Could you check a few things on this model? Use its own coordinates, in mm. A direction names the side the tool comes from. Round coordinates to 2 decimals unless told otherwise and drop trailing zeros. Write each loop counter-clockwise with the first axis right and the second up, starting at its lowest first coordinate (ties: lowest second). Pieces come first, ordered by that corner, then holes. Notation, with made-up numbers: (43.5, 49) -> (62.5, 49) arc R8 cw to (62.5, 59) -> close; hole circle Ø1 at (43, -9). An arc over 180 degrees is marked (long way). Answer as CSV lines item,"result". Start each with the question number.
Q1. Imagine slicing it at A-A on x = -4.5. Please give me the cut outline in (y, z).
Q2. For faces 1 (the flat face through (-2.932, -0.393, 2.761)), 2 (the cylindrical face through (-3.3, 1.41, -15.44)), 3 (the flat face through (0, 0.9, 3)), 4 (the flat face through (0, -0.9, 3)), 5 (the flat face through (0, 1.95, -15)), which set-ups out of +Z, -Z, +X, -X, +Y, -Y let a thin tool reach every point of the face, with its end or its side?
Q3. Imagine slicing it at B-B on y = 3. Please give me the cut outline in (x, z).
Q4. Will these pins go through, and if not, where does the flat tip stop? pin 1 Ø1.5 at (x, y) = (-4.5, -3) entering from +Z; pin 2 Ø2.5 at (x, z) = (0.5, -15) entering from +Y.
Q5. If I drill on line 1 (X direction, y = 0.5, z = 0.5) (3 decimals); line 2 (Z direction, x = -4, y = 0); line 3 (Y direction, x = -2, z = 3), over which ranges is the centre line in solid material (lowest first)? Write a range as [from, to].
from build123d import *

# Parameters (mm, degrees)
SKETCH1_W           = 11
SKETCH1_H           = 8.5
BOSS_EXTRUDE1_DEPTH = 14
SKETCH2_W           = 7.75
SKETCH2_H           = 3.9
BOSS_EXTRUDE2_DEPTH = 2.85
SKETCH4_W           = 6.85
SKETCH4_H           = 1.8
BOSS_EXTRUDE4_DEPTH = 5.6
FILLET6_R           = 0.3
CHAMFER1_SIZE       = 1
CUT_EXTRUDE1_DEPTH  = 0.15
CIRPATTERN1_COUNT   = 2
FILLET1_R           = 1.9
FILLET3_R           = 0.75
FILLET4_R           = 0.75


with BuildPart() as part:
    # Sketch1 → Boss-Extrude1 (new body)
    with BuildSketch(Plane.XY):
        Rectangle(SKETCH1_W, SKETCH1_H)
    extrude(amount=-BOSS_EXTRUDE1_DEPTH)

    # Sketch2 → Boss-Extrude2 (add)
    with BuildSketch(Plane(origin=(0, 0, -14), x_dir=(-1, 0, 0), z_dir=(0, 0, -1))):
        Rectangle(SKETCH2_W, SKETCH2_H)
    extrude(amount=BOSS_EXTRUDE2_DEPTH)

    # Sketch4 → Boss-Extrude4 (add)
    with BuildSketch(Plane.XY):
        Rectangle(SKETCH4_W, SKETCH4_H)
    extrude(amount=BOSS_EXTRUDE4_DEPTH)

    # Fillet6
    fillet6_edges = [part.edges().sort_by_distance(p)[0] for p in [
        (3.425, 0.9, 2.8),
        (-3.425, 0.9, 2.8),
    ]]
    fillet(fillet6_edges, radius=FILLET6_R)

    # Chamfer1
    chamfer1_edges = [part.edges().sort_by_distance(p)[0] for p in [
        (3.425, -0.9, 2.8),
        (-3.425, -0.9, 2.8),
    ]]
    chamfer(chamfer1_edges, length=CHAMFER1_SIZE)

    # Sketch5 → Cut-Extrude1 (cut)
    with BuildSketch(Plane.XZ.offset(4.25)):
        with BuildLine():
            Line((0, -3.279495805), (-0.485840634, -4.214842566))
            Line((-0.485840634, -4.214842566), (-0.093629021, -4.214842566))
            Line((-0.093629021, -4.214842566), (-0.093629021, -7.363659965))
            Line((-0.093629021, -7.363659965), (-1.035027967, -6.623865099))
            ThreePointArc((-1.035027967, -6.623865099), (-1.082535613, -6.564943154), (-1.099509752, -6.491182388))
            Line((-1.099509752, -6.491182388), (-1.099509752, -6.225332236))
            ThreePointArc((-1.099509752, -6.225332236), (-1.214270304, -5.348067145), (-1.329030856, -6.225332236))
            Line((-1.329030856, -6.225332236), (-1.329030856, -6.428798928))
            ThreePointArc((-1.329030856, -6.428798928), (-1.278108438, -6.650081225), (-1.135585502, -6.82684706))
            Line((-1.135585502, -6.82684706), (-0.158110806, -7.59499192))
            ThreePointArc((-0.158110806, -7.59499192), (-0.11060316, -7.653913865), (-0.093629021, -7.727674631))
            Line((-0.093629021, -7.727674631), (-0.093629021, -8.098323238))
            ThreePointArc((-0.093629021, -8.098323238), (0, -9.291083784), (0.093629021, -8.098323238))
            Line((0.093629021, -8.098323238), (0.093629021, -7.087908213))
            ThreePointArc((0.093629021, -7.087908213), (0.116268533, -7.003479025), (0.178112432, -6.941703889))
            Line((0.178112432, -6.941703889), (1.273368459, -6.310440139))
            ThreePointArc((1.273368459, -6.310440139), (1.458900155, -6.12511473), (1.526818691, -5.871827167))
            Line((1.526818691, -5.871827167), (1.526818691, -5.55143287))
            Line((1.526818691, -5.55143287), (1.774241614, -5.55143287))
            Line((1.774241614, -5.55143287), (1.774241614, -4.840448102))
            Line((1.774241614, -4.840448102), (1.063256846, -4.840448102))
            Line((1.063256846, -4.840448102), (1.063256846, -5.55143287))
            Line((1.063256846, -5.55143287), (1.321069322, -5.55143287))
            Line((1.321069322, -5.55143287), (1.321069322, -5.935219876))
            ThreePointArc((1.321069322, -5.935219876), (1.29842981, -6.019649064), (1.236585912, -6.081424201))
            Line((1.236585912, -6.081424201), (0.093629021, -6.740180906))
            Line((0.093629021, -6.740180906), (0.093629021, -4.214842566))
            Line((0.093629021, -4.214842566), (0.485840634, -4.214842566))
            Line((0.485840634, -4.214842566), (0, -3.279495805))
        make_face()
    cut_extrude1 = extrude(amount=-CUT_EXTRUDE1_DEPTH, mode=Mode.SUBTRACT)

    # CirPattern1: Cut-Extrude1 ×2 about axis
    cirpattern1_axis = Axis((0, 0, 0), (0, 0, 1))
    for i in range(1, CIRPATTERN1_COUNT):
        add(cut_extrude1.rotate(cirpattern1_axis, i * 360 / CIRPATTERN1_COUNT), mode=Mode.SUBTRACT)

    # Fillet1
    fillet1_edges = [part.edges().sort_by_distance(p)[0] for p in [
        (3.875, 1.95, -15.425),
        (3.875, -1.95, -15.425),
        (-3.875, -1.95, -15.425),
        (-3.875, 1.95, -15.425),
    ]]
    fillet(fillet1_edges, radius=FILLET1_R)

    # Fillet3
    fillet3_edges = [part.edges().sort_by_distance(p)[0] for p in [
        (5.5, -4.25, -7),
        (-5.5, -4.25, -7),
        (-5.5, 4.25, -7),
        (5.5, 4.25, -7),
    ]]
    fillet(fillet3_edges, radius=FILLET3_R)

    # Fillet4
    fillet4_edges = [part.edges().sort_by_distance(p)[0] for p in [
        (0, -4.25, -14),
        (5.5, 0, -14),
        (-5.5, 0, -14),
        (0, 4.25, -14),
        (5.280330086, 4.030330086, -14),
        (-5.280330086, 4.030330086, -14),
        (-5.280330086, -4.030330086, -14),
        (5.280330086, -4.030330086, -14),
    ]]
    fillet(fillet4_edges, radius=FILLET4_R)


solid = part.part
Checks:
1,outline,"(-4.25, -13.25) arc R0.75 ccw to (-3.5, -14) -> (3.5, -14) arc R0.75 ccw to (4.25, -13.25) -> (4.25, 0) -> (-4.25, 0) -> close"
2,face 1,"+Z, -X, -Y"
2,face 2,"-Z, -X, +Y"
2,face 3,"+Z, +X, -X, +Y"
2,face 4,"+Z, +X, -X, -Y"
2,face 5,"-Z, +X, -X, +Y"
3,outline,"(-5.5, -13.25) arc R0.75 ccw to (-4.75, -14) -> (4.75, -14) arc R0.75 ccw to (5.5, -13.25) -> (5.5, 0) -> (-5.5, 0) -> close"
4,pin 1,"z = 0"
4,pin 2,"y = 4.06"
5,line 1,"[-3.425, 3.425]"
5,line 2,"[-14, 0]"
5,line 3,"[-0.9, 0.9]"
